```python
from build123d import *

# Parameters (mm, degrees)
PAD_DEPTH       = 3.2
SKETCH007_R     = 1.7
POCKET003_DEPTH = 3.201
POCKET_DEPTH    = 3.201


with BuildPart() as part:
    # Sketch → Pad (new body)
    with BuildSketch(Plane.XY):
        with BuildLine():
            Line((-21, 45), (21, 45))
            ThreePointArc((25, 41), (23.828427, 43.828427), (21, 45))
            Line((25, 41), (25, -41))
            ThreePointArc((21, -45), (23.828427, -43.828427), (25, -41))
            Line((21, -45), (-21, -45))
            ThreePointArc((-25, -41), (-23.828427, -43.828427), (-21, -45))
            Line((-25, -41), (-25, 41))
            ThreePointArc((-21, 45), (-23.828427, 43.828427), (-25, 41))
        make_face()
    extrude(amount=PAD_DEPTH)

    # Sketch007 → Pocket003 (cut, through all)
    with BuildSketch(Plane.XY.offset(3.2)):
        with Locations((-19, 39)):
            Circle(SKETCH007_R)
        with Locations((19, 39)):
            Circle(SKETCH007_R)
        with Locations((-19, -39)):
            Circle(SKETCH007_R)
        with Locations((19, -39)):
            Circle(SKETCH007_R)
    extrude(amount=-POCKET003_DEPTH, mode=Mode.SUBTRACT)

    # Sketch001 (on Face9 of Pad) → Pocket (cut, through all)
    with BuildSketch(Plane(origin=(0, 0, 0), x_dir=(1, 0, 0), z_dir=(0, 0, -1))):
        with BuildLine():
            Line((-13, 36), (13, 36))
            ThreePointArc((16, 33), (15.12132, 35.12132), (13, 36))
            Line((16, 33), (16, -33))
            ThreePointArc((13, -36), (15.12132, -35.12132), (16, -33))
            Line((13, -36), (-13, -36))
            ThreePointArc((-16, -33), (-15.12132, -35.12132), (-13, -36))
            Line((-16, -33), (-16, 33))
            ThreePointArc((-13, 36), (-15.12132, 35.12132), (-16, 33))
        make_face()
    extrude(amount=-POCKET_DEPTH, mode=Mode.SUBTRACT)


solid = part.part
```
Geometry check sheet. Reference: the model listing, model coordinates, mm. A direction names the side the tool comes from. Coordinates: 2 decimals unless noted, no trailing zeros. Loops run counter-clockwise (first coordinate to the right, second up) from the corner with the lowest first, then second, coordinate; pieces in that order, holes last. Notation, with made-up numbers: (55.25, 23) -> (91.25, 23) arc R30 cw to (91.25, 61) -> close; hole circle Ø9 at (47.25, 5.5). An arc over 180 degrees is marked (long way). Put each result on its own line as item: value.
1) Cross-section at D-D on x = -5. Record the boundary of the cut face in (y, z), plus the area to 3 significant figures.
Result set:
outline: (-45, 0) -> (-36, 0) -> (-36, 3.2) -> (-45, 3.2) -> close; (36, 0) -> (45, 0) -> (45, 3.2) -> (36, 3.2) -> close
area: 57.6 mm^2
2) Tool access check on faces 4 (the flat face through (0, -45, 2)), 5 (the cylindrical face through (15.14, -35.1, 1.58)). Record the directions out of +Z, -Z, +X, -X, +Y, -Y that give a thin tool (end or side, any length) a straight path to the whole face; none if there is none.
Result set:
face 4: +Z, -Z, +X, -X, -Y
face 5: +Z, -Z
3) Cross-section at A-A on x = 19. Record the boundary of the cut face in (y, z), plus the area to 3 significant figures.
Result set:
outline: (-45, 0) -> (-40.7, 0) -> (-40.7, 3.2) -> (-45, 3.2) -> close; (-37.3, 0) -> (37.3, 0) -> (37.3, 3.2) -> (-37.3, 3.2) -> close; (40.7, 0) -> (45, 0) -> (45, 3.2) -> (40.7, 3.2) -> close
area: 266 mm^2
4) Release check for a two-part mould opening along X. For faces 1 (the cylindrical face through (23.797, -43.859, 1.578)), 2 (the flat face through (0, -36, 2)), 3 (the flat face through (17, 1, 3.2)) record: released by +X, released by -X, zero draft, split by the parting line, or undercut.
Result set:
face 1: released by +X
face 2: undercut
face 3: zero draft
5) Thickness scan on line 1 (Y direction, x = 19, z = 0.9); line 2 (Y direction, x = 7.5, z = 2.25); line 3 (X direction, y = 10.5, z = 1.65). Record the ranges inside material, lowest first.
Result set:
line 1: y = -45 to -40.7, -37.3 to 37.3, 40.7 to 45
line 2: y = -45 to -36, 36 to 45
line 3: x = -25 to -16, 16 to 25
6) Cross-section at B-B on z = 1.05. Record the boundary of the cut face in (x, y).
Result set:
outline: (-25, -41) arc R4 ccw to (-21, -45) -> (21, -45) arc R4 ccw to (25, -41) -> (25, 41) arc R4 ccw to (21, 45) -> (-21, 45) arc R4 ccw to (-25, 41) -> close; hole circle Ø3.4 at (-19, -39); hole circle Ø3.4 at (-19, 39); hole (-16, -33) arc R3 ccw to (-13, -36) -> (13, -36) arc R3 ccw to (16, -33) -> (16, 33) arc R3 ccw to (13, 36) -> (-13, 36) arc R3 ccw to (-16, 33) -> close; hole circle Ø3.4 at (19, -39); hole circle Ø3.4 at (19, 39)
7) Cross-section at C-C on y = 26. Record the boundary of the cut face in (x, z).
Result set:
outline: (-25, 0) -> (-16, 0) -> (-16, 3.2) -> (-25, 3.2) -> close; (16, 0) -> (25, 0) -> (25, 3.2) -> (16, 3.2) -> close
